Could you check a few things on this drawing? It's one solid part, dimensions in mm from its lowest x, y, z. Round coordinates to 2 decimals unless told otherwise and drop trailing zeros. Order: outer loops, then holes, each group sorted by start corner. A loop starts at its lowest first (then second) coordinate and runs counter-clockwise, first axis right, second up. Notation, with made-up numbers: (66.5, 28.5) - (73.5, 28.5) arc R23 cw to (73.5, 49.5) - close; hole circle Ø4 at (23.25, 57.5). An arc over 180 degrees is marked (long way). Use one line per item in the form item = value.
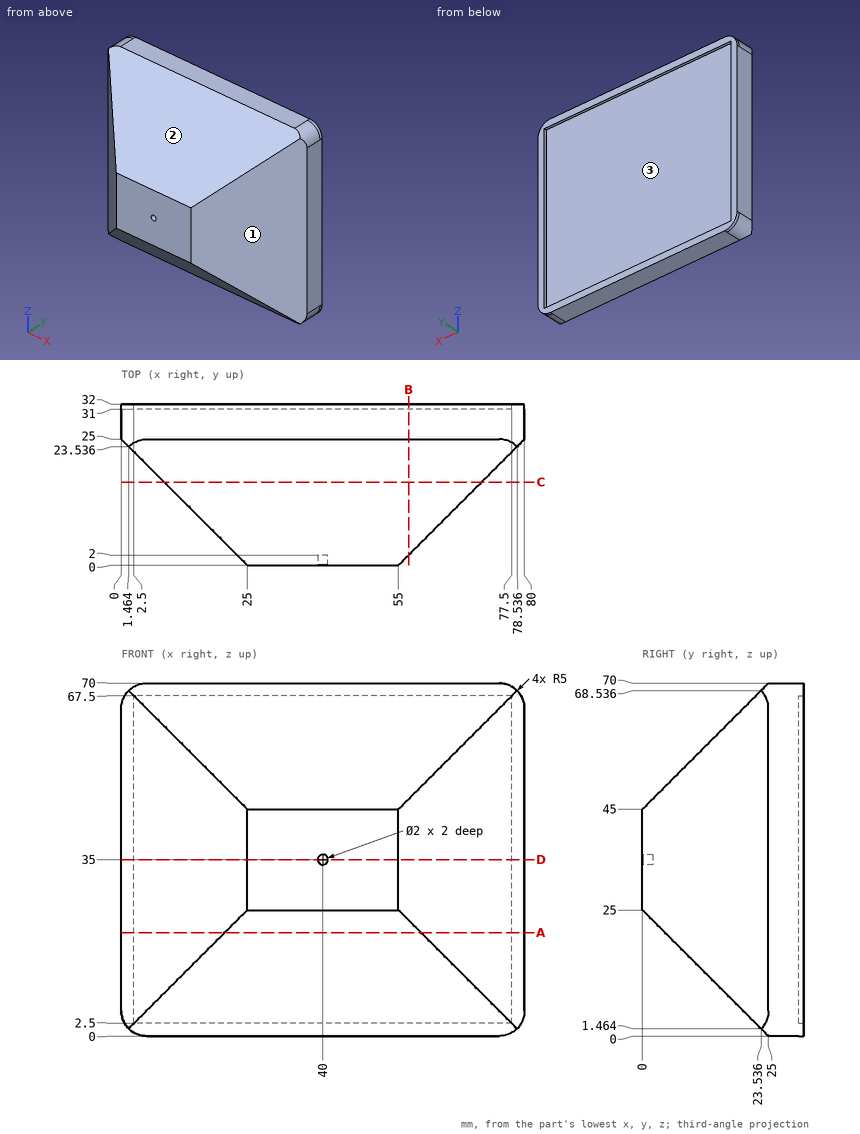
Item 1: Imagine slicing it at B-B on x = 57. Please give me the cut outline in (y, z).
Found:
outline = (2, 23) - (25, 0) - (32, 0) - (32, 2.5) - (31, 2.5) - (31, 67.5) - (32, 67.5) - (32, 70) - (25, 70) - (2, 47) - close
Item 2: Imagine slicing it at A-A on z = 20.5. Please give me the cut outline in (x, y).
Found:
outline = (0, 25) - (20.5, 4.5) - (59.5, 4.5) - (80, 25) - (80, 32) - (77.5, 32) - (77.5, 31) - (2.5, 31) - (2.5, 32) - (0, 32) - close
Item 3: I need wall thicknesses on L1, parallel to Y at x = 22.5, z = 30.5; L2, parallel to Z at x = 40, y = 1.4; L3, parallel to Z at x = 40, y = 1.25. Which ranges of each line are inside material? Lowest first, please.
Found:
L1 = 2.5 to 31
L2 = 23.6 to 34, 36 to 46.4
L3 = 23.75 to 34, 36 to 46.25
Item 4: Imagine slicing it at C-C on y = 16.5. Please give me the cut outline in (x, z), plus the area to 3 significant figures.
Found:
outline = (8.5, 8.5) - (71.5, 8.5) - (71.5, 61.5) - (8.5, 61.5) - close
area = 3,340 mm2
Item 5: Will these pins go through, and if not, where does the flat tip stop? P1, Ø3, axis at x = 49.5, y = 14.5, coming from the -Z side; P2, Ø3, axis at x = 56, y = 20.5, coming from the -Z side; P3, Ø1.5, axis at x = 60.5, z = 26.5, coming from the -Y side.
Found:
P1 = 9
P2 = 3
P3 = 4.75
Item 6: Imagine slicing it at D-D on z = 35. Please give me the cut outline in (x, y).
Found:
outline = (0, 25) - (25, 0) - (39, 0) - (39, 2) - (41, 2) - (41, 0) - (55, 0) - (80, 25) - (80, 32) - (77.5, 32) - (77.5, 31) - (2.5, 31) - (2.5, 32) - (0, 32) - close
Item 7: If we mould it in two halves opening along Z, with no side actions, what happens to the marked faces 1, 2 and 3? For each: released by +Z, released by -Z, zero draft, split by the parting line, or undercut.
Found:
face_1 = zero draft
face_2 = released by +Z
face_3 = undercut
